Source: CAD feature listing. Evaluate the final solid. Frame: model axes, mm. Face numbers are marked on the shaded views. A direction names the side the tool comes from. Give positions to 0.01 mm unless a question says otherwise; leave off trailing zeros. Loops run counter-clockwise (first coordinate to the right, second up) from the corner with the lowest first, then second, coordinate; pieces in that order, holes last. Notation, with made-up numbers: M -1,21 L 20,21 A30 cw 20,58 Z; hole C 15.5,80 d6. An arc over 180 degrees is marked long. Answer in a Markdown table with one row per item.
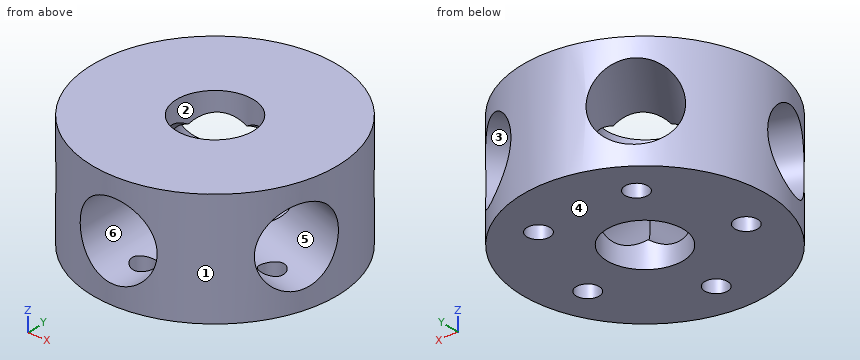
```python
from build123d import *

# Parameters (mm, degrees)
SKETCH1_R           = 32
SKETCH1_R_2         = 10
BOSS_EXTRUDE1_DEPTH = 15
SKETCH2_R           = 10
CUT_EXTRUDE1_DEPTH  = 48.675989764
CIRPATTERN1_COUNT   = 5
SKETCH4_R           = 3
CUT_EXTRUDE3_DEPTH  = 11
CIRPATTERN2_COUNT   = 5


with BuildPart() as part:
    # Sketch1 → Boss-Extrude1 (new, symmetric)
    with BuildSketch(Plane.XY):
        Circle(SKETCH1_R)
        Circle(SKETCH1_R_2, mode=Mode.SUBTRACT)
    extrude(amount=BOSS_EXTRUDE1_DEPTH, both=True)

    # Sketch2 → Cut-Extrude1 (cut, through all)
    with BuildSketch(Plane(origin=(0, 0, 0), x_dir=(1, 0, 0), z_dir=(0, 1, 0))):
        with Locations(Location((0, 0, 0), (0, 0, 270))):
            Circle(SKETCH2_R)
    cut_extrude1 = extrude(amount=-CUT_EXTRUDE1_DEPTH, mode=Mode.SUBTRACT)

    # CirPattern1: Cut-Extrude1 ×5 about axis
    cirpattern1_axis = Axis((0, 0, 15), (0, 0, -1))
    for i in range(1, CIRPATTERN1_COUNT):
        add(cut_extrude1.rotate(cirpattern1_axis, i * 360 / CIRPATTERN1_COUNT), mode=Mode.SUBTRACT)

    # Sketch4 → Cut-Extrude3 (cut)
    with BuildSketch(Plane.XY.offset(-15)):
        with Locations(Location((-12.6186816, 18.021344974, 0), (0, 0, 180))):
            Circle(SKETCH4_R)
    cut_extrude3 = extrude(amount=CUT_EXTRUDE3_DEPTH, mode=Mode.SUBTRACT)

    # CirPattern2: Cut-Extrude3 ×5 about axis
    cirpattern2_axis = Axis((0, 0, 0), (0, 0, 1))
    for i in range(1, CIRPATTERN2_COUNT):
        add(cut_extrude3.rotate(cirpattern2_axis, i * 360 / CIRPATTERN2_COUNT), mode=Mode.SUBTRACT)


solid = part.part
```
1) Section A-A, the plane z = -6. Return loops of the section in (x, y).
Reply:
| item | result |
|---|---|
| outline | M -31.94,-1.97 L -12.94,4.21 L -24.68,20.36 A32 ccw Z; M -27,-17.18 A32 ccw -8,-30.98 L -8,-11.01 Z; M -11.74,29.77 L 0,13.61 L 11.74,29.77 A32 ccw Z; M 8,-30.98 A32 ccw 27,-17.18 L 8,-11.01 Z; M 12.94,4.21 L 31.94,-1.97 A32 ccw 24.68,20.36 Z |
2) Pull-direction query (X, two-part tool) for the marked faces 1, 2, 3 and 4; classes: released by +X, released by -X, zero draft, split by the parting line, or undercut.
Reply:
| item | result |
|---|---|
| face 1 | split by the parting line |
| face 2 | undercut |
| face 3 | undercut |
| face 4 | zero draft |
3) Section C-C, the plane x = -2. Count the separate pieces of the cut face and the enclosed holes in it, then the cut area to 3 significant figures.
Reply:
| item | result |
|---|---|
| separate pieces | 4 |
| enclosed holes | 0 |
| area | 738 mm² |
4) Section D-D, the plane z = 0. Return loops of the section in (x, y), then the cut area to 3 significant figures.
Reply:
| item | result |
|---|---|
| outline | M -32,0.12 L -16.18,5.26 L -25.96,18.71 A32 ccw Z; M -25.82,-18.9 A32 ccw -10,-30.4 L -10,-13.76 Z; M -9.78,30.47 L 0,17.01 L 9.78,30.47 A32 ccw Z; M 10,-30.4 A32 ccw 25.82,-18.9 L 10,-13.76 Z; M 16.18,5.26 L 32,0.12 A32 ccw 25.96,18.71 Z |
| area | 758 mm² |
5) Set-up query: the marked faces 5 and 6. Return all of +Z, -Z, +X, -X, +Y, -Y with unobstructed straight access to the full face (end or side cutting, diameter ignored); none if empty.
Reply:
| item | result |
|---|---|
| face 5 | none |
| face 6 | -Y |
6) Material intervals for L1, parallel to Y at x = 10, z = 8; L2, parallel to X at y = -5, z = -12.5; L3, parallel to Z at x = 1.5, y = 14, sorted ascending.
Reply:
| item | result |
|---|---|
| L1 | y = -30.4 to -9.56, 3.06 to 3.56, 23.97 to 30.4 |
| L2 | x = -31.61 to -23.67, -18.4 to -8.66, 8.66 to 18.72, 22.88 to 31.61 |
| L3 | z = -15 to -7.13, 7.13 to 15 |
7) Pin query (flat end, axial travel): pin 1 Ø3 at (y, z) = (21, 1) entering from +X; pin 2 Ø2 at (x, z) = (-23, -7.5) entering from +Y; pin 3 Ø12 at (x, z) = (-9, 9) entering from +Y. Return the tip coordinate at first contact, or that it passes through.
Reply:
| item | result |
|---|---|
| pin 1 | stops at x = 4.07 |
| pin 2 | stops at y = 22.42 |
| pin 3 | stops at y = 31.86 |
8) Section B-B, the plane z = -12. Return loops of the section in (x, y), then the cut area to 3 significant figures.
Reply:
| item | result |
|---|---|
| outline | C 0,0 d64; hole C -21.04,-6.43 d6; hole C -12.62,18.02 d6; hole C 0,0 d20; hole C -0.38,-22 d6; hole C 13.24,17.57 d6; hole C 20.8,-7.16 d6 |
| area | 2,760 mm² |
